Source: CAD feature listing. Evaluate the final solid. Frame: model axes, mm. Face numbers are marked on the shaded views. A direction names the side the tool comes from. Give positions to 0.01 mm unless a question says otherwise; leave off trailing zeros. Loops run counter-clockwise (first coordinate to the right, second up) from the corner with the lowest first, then second, coordinate; pieces in that order, holes last. Notation, with made-up numbers: M 48.5,-22.75 L 98.5,-22.75 A12 cw 98.5,-13.75 Z; hole C 66,85 d9. An arc over 180 degrees is marked long. Write item = value, one per line.
from build123d import *

# Parameters (mm, degrees)
SKETCH1_W                  = 20
SKETCH1_H                  = 22
BOSS_EXTRUDE1_DEPTH        = 12
HOLE1_D                    = 4.92
HOLE1_DEPTH                = 11
HOLE1_TIP                  = 1.478117123
M3_5_CLEARANCE_HOLE1_D     = 4.13
M3_5_CLEARANCE_HOLE1_DEPTH = 12
M3_5_CLEARANCE_HOLE1_TIP   = 1.240777178
CHAMFER1_SIZE              = 0.25


with BuildPart() as part:
    # Sketch1 → Boss-Extrude1 (new body)
    with BuildSketch(Plane(origin=(0, 0, 0), x_dir=(0, 0, -1), z_dir=(1, 0, 0))):
        with Locations((10, 11)):
            Rectangle(SKETCH1_W, SKETCH1_H)
    extrude(amount=-BOSS_EXTRUDE1_DEPTH)

    # Hole1
    with Locations(Plane(origin=(0, 0, -20), x_dir=(-1, 0, 0), z_dir=(0, 0, -1))):
        with Locations((6, 17)):
            Hole(HOLE1_D / 2, depth=HOLE1_DEPTH)
            with Locations((0, 0, -(HOLE1_DEPTH + HOLE1_TIP / 2))):  # 118° drill point
                Cone(0, HOLE1_D / 2, HOLE1_TIP, mode=Mode.SUBTRACT)

    # M3.5 Clearance Hole1
    with Locations(Plane(origin=(0, 0, 0), x_dir=(-1, 0, 0), z_dir=(0, -1, 0))):
        with Locations((6, 16), (6, 6)):
            Hole(M3_5_CLEARANCE_HOLE1_D / 2, depth=M3_5_CLEARANCE_HOLE1_DEPTH)
            with Locations((0, 0, -(M3_5_CLEARANCE_HOLE1_DEPTH + M3_5_CLEARANCE_HOLE1_TIP / 2))):  # 118° drill point
                Cone(0, M3_5_CLEARANCE_HOLE1_D / 2, M3_5_CLEARANCE_HOLE1_TIP, mode=Mode.SUBTRACT)

    # Chamfer1
    chamfer1_edges = [part.edges().sort_by_distance(p)[0] for p in [
        (-12, 11, -20),
        (-12, 22, -10),
        (-12, 11, 0),
        (0, 22, -10),
        (0, 11, -20),
        (0, 0, -10),
        (0, 11, 0),
        (-6, 22, 0),
        (-6, 22, -20),
        (-6, 0, -20),
        (-6, 0, 0),
        (-12, 0, -10),
    ]]
    chamfer(chamfer1_edges, length=CHAMFER1_SIZE)


solid = part.part
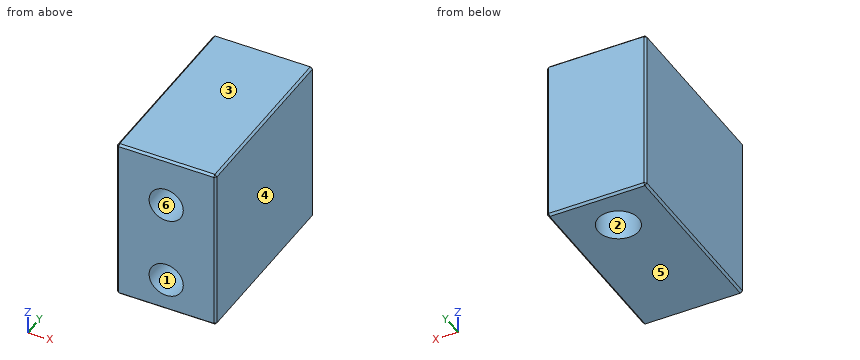
1. Cut plane B-B, the plane y = 4. Return the cut outline in (x, z) (3 decimals), then the cut area to 3 significant figures.
Derived:
outline = M -12,-19.75 L -11.75,-20 L -0.25,-20 L 0,-19.75 L 0,-0.25 L -0.25,0 L -11.75,0 L -12,-0.25 Z; hole C -6,-16 d4.13; hole C -6,-6 d4.13
area = 213 mm²
2. Cut plane A-A, the plane z = -12. Return the cut outline in (x, y).
Derived:
outline = M -12,0.25 L -11.75,0 L -0.25,0 L 0,0.25 L 0,21.75 L -0.25,22 L -11.75,22 L -12,21.75 Z; hole C -6,17 d4.92
3. Material intervals for probe 1 along Z at (x, y) = (-6, 2.5) (3 decimals); probe 2 along Y at (x, z) = (-6, -18.5); probe 3 along X at (y, z) = (17, -17.5), sorted ascending. Write a range as from..to.
Derived:
probe_1 = -20..-18.065, -13.935..-8.065, -3.935..0
probe_2 = 0..14.54, 19.46..22
probe_3 = -12..-8.46, -3.54..0
4. Pull-direction query (Z, two-part tool) for the marked faces 4, 5 and 6; classes: +Z half, -Z half, draft (parallel to the pull), parting line (faces both ways), or undercut.
Derived:
face_4 = draft
face_5 = -Z half
face_6 = undercut
5. First-contact query: pin 1 Ø3.5 at (x, z) = (-6, -6) entering from -Y. Flat tip, straight axial feed; report the tip coordinate or a pass-through.
Derived:
pin_1 = 12.19
6. Reachability of the marked faces 1, 2 and 3 from +Z, -Z, +X, -X, +Y, -Y: full face, straight path, thin tool, end or side. Return the list, or none.
Derived:
face_1 = -Y
face_2 = -Z
face_3 = +Z, +X, -X, +Y, -Y
